from build123d import *

# Parameters (mm, degrees)
SKETCH_1_R          = 1.25
EXTRUDE_1_DEPTH     = 2
SKETCH_2_R          = 1
SKETCH_2_W          = 45
SKETCH_2_H          = 95.5
CUT_EXTRUDE_1_DEPTH = 74.159073258
EXTRUDE_1_2_DEPTH   = 2
FILLET_1_R          = 1
FILLET_2_R          = 1
FILLET_3_R          = 3


with BuildPart() as part:
    # 草图1 → Extrude 1 (new body)
    with BuildSketch(Plane(origin=(0, 0, 0), x_dir=(1, 0, 0), z_dir=(0, 1, 0))):
        with BuildLine():
            Line((-28.5, 31.30958424), (-28.5, 9))
            Line((-28.5, 9), (-31.5, 9))
            Line((-31.5, 9), (-31.5, -6))
            Line((-31.5, -6), (-28.5, -6))
            Line((-28.5, -6), (-28.5, -31.30958424))
            ThreePointArc((-28.5, -31.30958424), (-28.740401367, -32.486281051), (-29.423076923, -33.474391514))
            ThreePointArc((-29.423076923, -33.474391514), (-30.5, -36), (-29.423076923, -38.525608486))
            ThreePointArc((-29.423076923, -38.525608486), (-28.740401367, -39.513718949), (-28.5, -40.69041576))
            Line((-28.5, -40.69041576), (-28.5, -46))
            Line((-28.5, -46), (-31.5, -46))
            Line((-31.5, -46), (-31.5, -61))
            Line((-31.5, -61), (-28.5, -61))
            Line((-28.5, -61), (-28.5, -66))
            Line((-28.5, -66), (28.5, -66))
            Line((28.5, -66), (28.5, -61))
            Line((28.5, -61), (31.5, -61))
            Line((31.5, -61), (31.5, -46))
            Line((31.5, -46), (28.5, -46))
            Line((28.5, -46), (28.5, -40.69041576))
            ThreePointArc((28.5, -40.69041576), (28.740401367, -39.513718949), (29.423076923, -38.525608486))
            ThreePointArc((29.423076923, -38.525608486), (30.5, -36), (29.423076923, -33.474391514))
            ThreePointArc((29.423076923, -33.474391514), (28.740401367, -32.486281051), (28.5, -31.30958424))
            Line((28.5, -31.30958424), (28.5, -6))
            Line((28.5, -6), (31.5, -6))
            Line((31.5, -6), (31.5, 9))
            Line((31.5, 9), (28.5, 9))
            Line((28.5, 9), (28.5, 31.30958424))
            ThreePointArc((28.5, 31.30958424), (28.740401367, 32.486281051), (29.423076923, 33.474391514))
            ThreePointArc((29.423076923, 33.474391514), (30.247278068, 37.305827381), (27, 39.5))
            Line((27, 39.5), (-27, 39.5))
            ThreePointArc((-27, 39.5), (-30.247278068, 37.305827381), (-29.423076923, 33.474391514))
            ThreePointArc((-29.423076923, 33.474391514), (-28.740401367, 32.486281051), (-28.5, 31.30958424))
        make_face()
        with Locations(Location((-27, 36, 0), (0, 0, 270))):
            Circle(SKETCH_1_R, mode=Mode.SUBTRACT)
        with Locations(Location((-27, -36, 0), (0, 0, 90))):
            Circle(SKETCH_1_R, mode=Mode.SUBTRACT)
        with Locations(Location((27, 36, 0), (0, 0, 90))):
            Circle(SKETCH_1_R, mode=Mode.SUBTRACT)
        with Locations(Location((27, -36, 0), (0, 0, 270))):
            Circle(SKETCH_1_R, mode=Mode.SUBTRACT)
    extrude(amount=EXTRUDE_1_DEPTH)

    # 草图2 → 切除-拉伸1 (cut, through all)
    with BuildSketch(Plane(origin=(0, 2, 0), x_dir=(1, 0, 0), z_dir=(0, 1, 0))):
        with Locations((-28.5, -45)):
            Circle(SKETCH_2_R)
        with Locations((-28.5, -62)):
            Circle(SKETCH_2_R)
        with Locations((28.5, -62)):
            Circle(SKETCH_2_R)
        with Locations((28.5, -45)):
            Circle(SKETCH_2_R)
        with Locations((-28.5, 10)):
            Circle(SKETCH_2_R)
        with Locations((-28.5, -7)):
            Circle(SKETCH_2_R)
        with Locations((28.5, -7)):
            Circle(SKETCH_2_R)
        with Locations((28.5, 10)):
            Circle(SKETCH_2_R)
        with Locations((0, -13.25)):
            Rectangle(SKETCH_2_W, SKETCH_2_H)
    extrude(amount=-CUT_EXTRUDE_1_DEPTH, mode=Mode.SUBTRACT)

    # 草图3 → Extrude 1 2 (add)
    # profile 1 of 3: a face of its own
    with BuildSketch(Plane(origin=(0, 2, 0), x_dir=(1, 0, 0), z_dir=(0, 1, 0))):
        Polygon((-24.083056856, 33.754056979), (20.916943144, -61.745943021), (24.083056856, -60.254056979), (-20.916943144, 35.245943021), align=None)
    # profile 2 of 3: a face of its own
    with BuildSketch(Plane(origin=(0, 2, 0), x_dir=(1, 0, 0), z_dir=(0, 1, 0))):
        Polygon((-20.916943144, -61.745943021), (24.083056856, 33.754056979), (20.916943144, 35.245943021), (-24.083056856, -60.254056979), align=None)
    # profile 3 of 3: a face of its own
    with BuildSketch(Plane(origin=(0, 2, 0), x_dir=(1, 0, 0), z_dir=(0, 1, 0))):
        Polygon((0, 38.60554146), (-24.434548332, -13.25), (0, -65.10554146), (24.434548332, -13.25), align=None)
        Polygon((0, 30.39445854), (-20.565451668, -13.25), (0, -56.89445854), (20.565451668, -13.25), align=None, mode=Mode.SUBTRACT)
    extrude(amount=-EXTRUDE_1_2_DEPTH)

    # 圆角1
    fillet_1_edges = [part.edges().sort_by_distance(p)[0] for p in [
        (31.5, 1, -9),
        (31.5, 1, 6),
        (31.5, 1, 46),
        (31.5, 1, 61),
        (28.5, 1, 66),
        (-28.5, 1, 66),
        (-31.5, 1, 61),
        (-31.5, 1, 46),
        (-31.5, 1, 6),
        (-31.5, 1, -9),
    ]]
    fillet(fillet_1_edges, radius=FILLET_1_R)

    # 圆角2
    fillet_2_edges = [part.edges().sort_by_distance(p)[0] for p in [
        (-1.934548332, 1, 61),
        (1.934548332, 1, 61),
        (-20.565451668, 1, 61),
        (20.565451668, 1, 61),
        (22.5, 1, 17.35554146),
        (22.5, 1, 9.14445854),
        (22.5, 1, -30.39445854),
        (22.5, 1, 56.89445854),
        (-1.934548332, 1, -34.5),
        (1.934548332, 1, -34.5),
        (20.565451668, 1, -34.5),
        (-20.565451668, 1, -34.5),
        (-22.5, 1, 17.35554146),
        (-22.5, 1, 9.14445854),
        (-22.5, 1, 56.89445854),
        (-22.5, 1, -30.39445854),
        (-11.25, 1, -14.73054146),
        (11.25, 1, -14.73054146),
        (11.25, 1, 41.23054146),
        (-11.25, 1, 41.23054146),
        (-11.25, 1, -6.51945854),
        (0, 1, -30.39445854),
        (11.25, 1, 33.01945854),
        (0, 1, 9.14445854),
        (11.25, 1, -6.51945854),
        (0, 1, 17.35554146),
        (-11.25, 1, 33.01945854),
        (0, 1, 56.89445854),
    ]]
    fillet(fillet_2_edges, radius=FILLET_2_R)

    # 圆角3
    fillet_3_edges = [part.edges().sort_by_distance(p)[0] for p in [
        (-13.184548332, 1, 37.125),
        (-13.184548332, 1, -10.625),
        (13.184548332, 1, 37.125),
        (13.184548332, 1, -10.625),
        (-1.934548332, 1, 13.25),
        (9.315451668, 1, 37.125),
        (1.934548332, 1, 13.25),
        (9.315451668, 1, -10.625),
        (20.565451668, 1, 13.25),
        (-9.315451668, 1, -10.625),
        (-9.315451668, 1, 37.125),
        (-20.565451668, 1, 13.25),
    ]]
    fillet(fillet_3_edges, radius=FILLET_3_R)


solid = part.part
Model file for the job. Use its own axes, mm. A direction names the side the tool comes from. Give positions to 0.01 mm unless a question says otherwise; leave off trailing zeros. Order: outer loops, then holes, each group sorted by start corner. A loop starts at its lowest first (then second) coordinate and runs counter-clockwise, first axis right, second up. Notation, with made-up numbers: M 18.25,21.25 L 34.25,21.25 A22 cw 34.25,33.25 Z; hole C -29.5,57 d1. An arc over 180 degrees is marked long. Write item = value, one per line.
Q1. Drill centre lines: line 1 (X direction, y = 1.05, z = -36); line 2 (X direction, y = 0.95, z = -2); line 3 (Z direction, x = -4.5, y = 1.3). Where is each one in solid material? Low to high. Write a range as [from, to].
Derived:
line_1 = [-30.5, -28.25], [-25.75, 25.75], [28.25, 30.5]
line_2 = [-31.5, -22.5], [-17.25, -13.38], [-9.12, -5.25], [5.25, 9.12], [13.38, 17.25], [22.5, 31.5]
line_3 = [-39.5, -34.5], [-29.06, -20.84], [-0.41, 7.81], [18.69, 26.91], [47.34, 55.56], [61, 66]
Q2. Flat gauge pins, fed straight in: pin 1 (0.6 mm diameter, centred on x = -30, y = 1, fed in from -Z); pin 2 (1 mm diameter, centred on y = 1.5, z = -25.5, fed in from -X); pin 3 (1 mm diameter, centred on y = 1, z = -10, fed in from +X). Where does each tip first touch, or does it go through?
Derived:
pin_1 = -38.23
pin_2 = -28.5
pin_3 = 27.63
Q3. Tool access for faces 1 (the cylindrical face through (28.734, 0.986, -32.471)), 2 (the flat face through (-28.5, 1, 42)), 3 (the flat face through (-6.496, 1.014, 3.57)): list every direction of +Z, -Z, +X, -X, +Y, -Y with a clear straight run to the whole face (end or side of a thin tool).
Derived:
face_1 = +X, +Y, -Y
face_2 = -X, +Y, -Y
face_3 = +Y, -Y
Q4. Two-plate mould, pull along X, no slides. Class faces 4 (the flat face through (-30, 1, 61)), 5 (the cylindrical face through (27.76, 0.99, -35.01)), 6 (the flat face through (-31.5, 1, 53)): pulls with the +X half, pulls with the -X half, needs draft (parallel to the pull), parting line crosses it, or undercut.
Derived:
face_4 = needs draft
face_5 = undercut
face_6 = pulls with the -X half
Q5. Cut at A-A, the plane z = -36. List the corners of the cut face in (x, y), then the cut area to 3 significant figures.
Derived:
outline = M -30.5,0 L -28.25,0 L -28.25,2 L -30.5,2 Z; M -25.75,0 L 25.75,0 L 25.75,2 L -25.75,2 Z; M 28.25,0 L 30.5,0 L 30.5,2 L 28.25,2 Z
area = 112 mm2
Q6. Cut at C-C, the plane z = 62. List the corners of the cut face in (x, y), then the cut area to 3 significant figures.
Derived:
outline = M -27.5,0 L 27.5,0 L 27.5,2 L -27.5,2 Z
area = 110 mm2
Q7. Cut at B-B, the plane y = 1.25. Count the separate pieces of the cut face and the enclosed holes in it, then the cut area to 3 significant figures.
Derived:
separate_pieces = 1
enclosed_holes = 16
area = 3,300 mm2
